Source: CAD feature listing. Evaluate the final solid. Frame: model axes, mm. Round coordinates to 2 decimals unless told otherwise and drop trailing zeros. Write each loop counter-clockwise with the first axis right and the second up, starting at its lowest first coordinate (ties: lowest second). Pieces come first, ordered by that corner, then holes. Notation, with made-up numbers: M 49,9.5 L 56,9.5 A19 ccw 56,44.5 Z; hole C -36.5,-19.5 d8. An arc over 180 degrees is marked long. Answer in a Markdown table with one row per item. Add a question column.
Item 1: Cut plane A-A on x = -21.5. Return loops of the section in (y, z), and give its area (4 significant figures).
Item 2: Cut plane D-D on y = 10.5. Return loops of the section in (x, z), and give its area (3 significant figures).
Item 3: Cut plane B-B on y = -22.5. Return loops of the section in (x, z), and give its area (3 significant figures).
Item 4: Mould query, pull axis Y, two halves, no side actions, for faces 1 (the face through (31.67, 26.34, 2.53)), 2 (the face through (38.49, 30.65, 2.54)), 3 (the face through (41.5, 0, 2)), 4 (the face through (-18.753, -22.379, 2.465)). Classes: released by +Y, released by -Y, zero draft, split by the parting line, or undercut.
Item 5: Contact query for flat-ended pins moving along their axis: pin 1 (3 mm diameter, centred on x = -17.5, y = 11, fed in from -Z); pin 2 (4.5 mm diameter, centred on x = 21.5, y = -22.5, fed in from +Z). Output: stop coordinate, or through.
Item 6: Cut plane C-C on z = 3.5. Return loops of the section in (x, y), and give its area (3 significant figures).
Item 7: Material intervals for probe 1 along X at (y, z) = (26.5, 0.25); probe 2 along Y at (x, z) = (21.5, 1.6); probe 3 along X at (y, z) = (13, 4.45), sorted ascending.
from build123d import *

# Parameters (mm, degrees)
SKETCH1_W            = 83
SKETCH1_H            = 67
BOSS_EXTRUDE1_DEPTH  = 5
M5_CLEARANCE_HOLE1_D = 5.5
M3_CLEARANCE_HOLE1_D = 3.4
SKETCH6_R            = 11.05
CUT_EXTRUDE1_DEPTH   = 6
FILLET1_R            = 10


with BuildPart() as part:
    # Sketch1 → Boss-Extrude1 (new body)
    with BuildSketch(Plane.XY):
        Rectangle(SKETCH1_W, SKETCH1_H)
    extrude(amount=BOSS_EXTRUDE1_DEPTH)

    # M5 Clearance Hole1 (through all)
    with Locations(Plane.XY.offset(5)):
        with Locations((21.5, -22.5), (-21.5, -22.5)):
            Hole(M5_CLEARANCE_HOLE1_D / 2)

    # M3 Clearance Hole1 (through all)
    with Locations(Plane(origin=(0, 0, 0), x_dir=(-1, 0, 0), z_dir=(0, 0, -1))):
        with Locations((-32.041076253, 28.00000478), (-1.041076253, 28.00000478), (-1.041076253, -2.99999522), (-32.041076253, -2.99999522)):
            Hole(M3_CLEARANCE_HOLE1_D / 2)

    # Sketch6 → Cut-Extrude1 (cut, through all)
    with BuildSketch(Plane.XY.offset(5)):
        with Locations((16.541076624, 12.500005008)):
            Circle(SKETCH6_R)
    extrude(amount=-CUT_EXTRUDE1_DEPTH, mode=Mode.SUBTRACT)

    # Fillet1
    fillet1_edges = [part.edges().sort_by_distance(p)[0] for p in [
        (41.5, -33.5, 2.5),
        (-41.5, -33.5, 2.5),
        (-41.5, 33.5, 2.5),
        (41.5, 33.5, 2.5),
    ]]
    fillet(fillet1_edges, radius=FILLET1_R)


solid = part.part
Results below:
| question | item | result |
|---|---|---|
| 1 | outline | M -33.5,0 L -25.25,0 L -25.25,5 L -33.5,5 Z; M -19.75,0 L 33.5,0 L 33.5,5 L -19.75,5 Z |
| 1 | area | 307.5 mm2 |
| 2 | outline | M -41.5,0 L 5.67,0 L 5.67,5 L -41.5,5 Z; M 27.41,0 L 41.5,0 L 41.5,5 L 27.41,5 Z |
| 2 | area | 306 mm2 |
| 3 | outline | M -41.5,0 L -24.25,0 L -24.25,5 L -41.5,5 Z; M -18.75,0 L 18.75,0 L 18.75,5 L -18.75,5 Z; M 24.25,0 L 41.5,0 L 41.5,5 L 24.25,5 Z |
| 3 | area | 360 mm2 |
| 4 | face 1 | undercut |
| 4 | face 2 | released by +Y |
| 4 | face 3 | zero draft |
| 4 | face 4 | undercut |
| 5 | pin 1 | z = 0 |
| 5 | pin 2 | through |
| 6 | outline | M -41.5,-23.5 A10 ccw -31.5,-33.5 L 31.5,-33.5 A10 ccw 41.5,-23.5 L 41.5,23.5 A10 ccw 31.5,33.5 L -31.5,33.5 A10 ccw -41.5,23.5 Z; hole C -21.5,-22.5 d5.5; hole C 1.04,-3 d3.4; hole C 1.04,28 d3.4; hole C 16.54,12.5 d22.1; hole C 21.5,-22.5 d5.5; hole C 32.04,-3 d3.4; hole C 32.04,28 d3.4 |
| 6 | area | 5,010 mm2 |
| 7 | probe 1 | -41.04 to 0.24, 1.84 to 31.24, 32.84 to 41.04 |
| 7 | probe 2 | -33.5 to -25.25, -19.75 to 2.63, 22.37 to 33.5 |
| 7 | probe 3 | -41.5 to 5.5, 27.58 to 41.5 |
